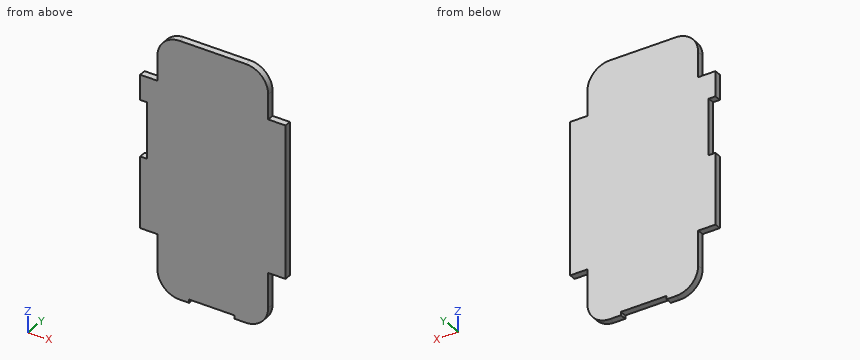
Autodesk Inventor part; units mm, degrees
ref_plane "YZ Plane" through (0, 0, 0) normal (1, 0, 0) x (0, 1, 0)
ref_plane "XZ Plane" through (0, 0, 0) normal (0, 1, 0) x (-1, 0, 0)
ref_plane "XY Plane" through (0, 0, 0) normal (0, 0, 1) x (1, 0, 0)
sketch "Sketch1" plane through (0, 0, 0) normal (0, 1, 0) x (-1, 0, 0)
  line L0 (49.6, -114.5) -> (49.6, -63.5)
  line L1 (49.6, -63.5) -> (65, -63.5)
  line L2 (-65, -63.5) -> (-49.6, -63.5)
  line L3 (-49.6, -63.5) -> (-49.6, -114.5)
  line L4 (-65, 72.3) -> (-49.6, 72.3)
  line L5 (-65, -63.5) -> (-65, 72.3)
  line L6 (-49.6, 72.3) -> (-49.6, 114.5)
  line L7 (49.6, 114.5) -> (49.6, 72.3)
  line L8 (49.6, 72.3) -> (65, 72.3)
  line L9 (49.6, 114.5) -> (-49.6, 114.5)
  line L10 (49.6, -114.5) -> (21.2, -114.5)
  line L11 (21.2, -114.5) -> (21.2, -111.5)
  line L12 (-49.6, -114.5) -> (-19.6, -114.5)
  line L13 (-19.6, -114.5) -> (-19.6, -111.5)
  line L14 (-19.6, -111.5) -> (21.2, -111.5)
  line L15 (65, 72.3) -> (65, 50)
  line L16 (65, 50) -> (59, 50)
  line L17 (59, 50) -> (59, 0)
  line L18 (59, 0) -> (65, 0)
  line L19 (65, 0) -> (65, -63.5)
  point P0 (0, 0)
  dimension "d3" = 51
  dimension "d5" = 15.4
  dimension "d8" = 15.4
  dimension "d10" = 42.2
  dimension "d11" = 28.4
  dimension "d13" = 30
  dimension "d14" = 3
  dimension "d15" = 40.8
  dimension "d16" = 22.3
  dimension "d17" = 6
  dimension "d18" = 50
extrude "Extrusion1" add sketch "Sketch1" along normal blind 6
fillet "Fillet1" radius 20 4 edges at (49.6, 3, -114.5) (-49.6, 3, -114.5) (49.6, 3, 114.5) (-49.6, 3, 114.5)
properties part number "kryt_v1,1"
Source: CAD feature listing. Evaluate the final solid. Frame: model axes, mm. Coordinates: 2 decimals unless noted, no trailing zeros. Write each loop counter-clockwise with the first axis right and the second up, starting at its lowest first coordinate (ties: lowest second). Pieces come first, ordered by that corner, then holes. Notation, with made-up numbers: (-34.5, 43) -> (-17.5, 43) arc R34 ccw to (-17.5, 73) -> close; hole circle Ø7 at (-12.75, -34). An arc over 180 degrees is marked (long way). Return JSON: item names as keys, results as strings. Group by question number.
1) Section query B-B, the plane z = -83. Return loops of the section in (x, y).
2) Section query C-C, the plane z = 44.5. Return loops of the section in (x, y).
3) Ray query, line 1 along Z through (x, y) = (14, 4.35); line 2 along X through (y, z) = (5.35, 82.5); line 3 along Z through (x, y) = (58.5, 1.75). Return the intervals inside material, ascending.
4) Section query A-A, the plane y = 4.9. Return loops of the section in (x, z), plus the area to 3 significant figures.
5) Contact query for flat-ended pins moving along their axis: P1, Ø1.8, axis at y = 4, z = 23, coming from the -X side; P2, Ø1.8, axis at x = 55.5, y = 2, coming from the +Z side; P3, Ø3, axis at x = -60, y = 2, coming from the -Z side. Output: stop coordinate, or through.
From the geometry:
{
 "1": {"outline": "(-49.6, 0) -> (49.6, 0) -> (49.6, 6) -> (-49.6, 6) -> close"},
 "2": {"outline": "(-59, 0) -> (65, 0) -> (65, 6) -> (-59, 6) -> close"},
 "3": {"line 1": "-111.5 to 114.5", "line 2": "-49.6 to 49.6", "line 3": "-63.5 to 72.3"},
 "4": {"outline": "(-65, -63.5) -> (-49.6, -63.5) -> (-49.6, -94.5) arc R20 ccw to (-29.6, -114.5) -> (-21.2, -114.5) -> (-21.2, -111.5) -> (19.6, -111.5) -> (19.6, -114.5) -> (29.6, -114.5) arc R20 ccw to (49.6, -94.5) -> (49.6, -63.5) -> (65, -63.5) -> (65, 72.3) -> (49.6, 72.3) -> (49.6, 94.5) arc R20 ccw to (29.6, 114.5) -> (-29.6, 114.5) arc R20 ccw to (-49.6, 94.5) -> (-49.6, 72.3) -> (-65, 72.3) -> (-65, 50) -> (-59, 50) -> (-59, 0) -> (-65, 0) -> close", "area": "26,100 mm²"},
 "5": {"P1": "x = -59", "P2": "z = 72.3", "P3": "z = -63.5"}
}
